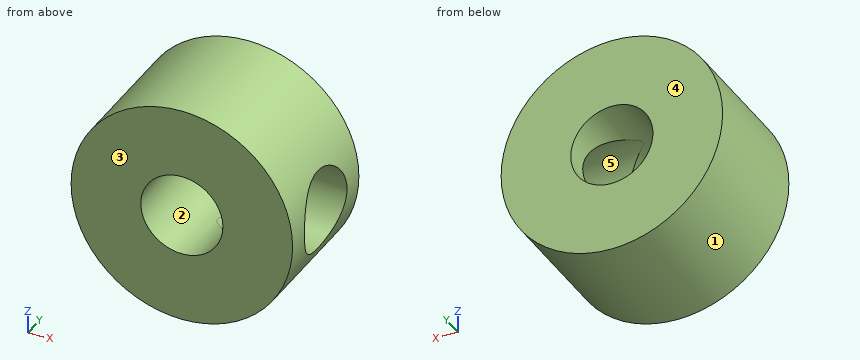
Autodesk Inventor part; units mm, degrees
ref_plane "Work Plane1" through (5.5182, 0, 0) normal (1, 0, 0) x (0, 1, 0)
ref_plane "XZ Plane" through (0, 0, 0) normal (0, 1, 0) x (-1, 0, 0)
ref_plane "XY Plane" through (0, 0, 0) normal (0, 0, 1) x (1, 0, 0)
sketch "Sketch1" plane through (0, 0, 0) normal (0, 1, 0) x (-1, 0, 0)
  circle A0 centre (0, 0) radius 5.5182
  dimension "d0" = 11.0363
extrude "Extrusion1" add sketch "Sketch1" along normal blind 6.3779
sketch "Sketch2" plane through (0, 6.3779, 0) normal (0, 1, 0) x (1, 0, 0)
  circle A0 centre (0, 0) radius 2.046
  dimension "d3" = 4.0919
extrude "Extrusion2" cut sketch "Sketch2" against normal blind 11.1125
ref_plane "Work Plane1" through (5.5182, 0, 0) normal (1, 0, 0) x (0, 1, 0)
sketch "Sketch3" plane through (5.5182, 0, 0) normal (1, 0, 0) x (0, 1, 0)
  line L0 (6.3779, -5.5182) -> (6.3779, 5.5182)
  line L1 (6.3779, 0) -> (0, 0)
  circle A0 centre (3.189, 0) radius 2.0472
  dimension "d6" = 4.0945
extrude "Extrusion3" cut sketch "Sketch3" against normal blind 5.3975
properties part number "Axle hub with no cricle thing"
The model under review builds one solid part; all positions refer to its coordinate system, in mm. Face numbers are marked on the shaded views. A direction names the side the tool comes from. Coordinates: 2 decimals unless noted, no trailing zeros. Write each loop counter-clockwise with the first axis right and the second up, starting at its lowest first coordinate (ties: lowest second). Pieces come first, ordered by that corner, then holes. Notation, with made-up numbers: (-4, 38) - (45, 38) arc R24 ccw to (45, 74) - close; hole circle Ø2 at (-33.5, 58.5). An arc over 180 degrees is marked (long way). Answer as CSV lines item,"result".
(1) We need section B-B (x = 1.5). Give the boundary of the cut face in (y, z), plus the area to 3 significant figures.
Data:
outline,"(0, -5.31) - (6.38, -5.31) - (6.38, -1.39) - (4.69, -1.39) arc R2.05 cw to (1.69, -1.39) - (0, -1.39) - close; (0, 1.39) - (1.69, 1.39) arc R2.05 cw to (4.69, 1.39) - (6.38, 1.39) - (6.38, 5.31) - (0, 5.31) - close"
area,"47.3 mm2"
(2) We need section C-C (y = 5.75). Give the boundary of the cut face in (x, z).
Data:
outline,"circle Ø11.04 at (0, 0); hole circle Ø4.09 at (0, 0)"
(3) Tool access review of the marked faces 4 and 5: name each direction out of +Z, -Z, +X, -X, +Y, -Y from which nothing blocks a thin tool from reaching the whole face with its end or side.
Data:
face 4,"+Z, -Z, +X, -X, +Y"
face 5,"+X"
(4) We need section D-D (x = 4). Give the boundary of the cut face in (y, z), plus the area to 3 significant figures.
Data:
outline,"(0, -3.8) - (6.38, -3.8) - (6.38, 3.8) - (0, 3.8) - close; hole circle Ø4.09 at (3.19, 0)"
area,"35.3 mm2"
(5) Clearance check with flat-ended pins moving along their axes: pin 1 Ø1 at (y, z) = (4, 3.5) entering from -X; pin 2 Ø1 at (x, y) = (3, 3.5) entering from -Z. State where each tip first meets the part, or that it passes through.
Data:
pin 1,"stops at x = -4.63"
pin 2,"stops at z = -4.92"
(6) For line 1 along Z through (x, y) = (0, 4.75); line 2 along Y through (x, z) = (4, 0); line 3 along X through (y, z) = (1, -0.75), list the stretches that pass through material, from the lowest coordinate up. Write a range as [from, to].
Data:
line 1,"z = [-5.52, -2.05], [2.05, 5.52]"
line 2,"y = [0, 1.14], [5.24, 6.38]"
line 3,"x = [-5.47, -1.9], [1.9, 5.47]"
(7) We need section A-A (z = 0). Give the boundary of the cut face in (x, y).
Data:
outline,"(-5.52, 0) - (-2.05, 0) - (-2.05, 6.38) - (-5.52, 6.38) - close; (2.05, 0) - (5.52, 0) - (5.52, 1.14) - (2.05, 1.14) - close; (2.05, 5.24) - (5.52, 5.24) - (5.52, 6.38) - (2.05, 6.38) - close"
(8) Mouldability with a two-part tool opening along X and no side actions: class the marked faces 1, 2 and 3 as pulls with the +X half, pulls with the -X half, needs draft (parallel to the pull), parting line crosses it, or undercut.
Data:
face 1,"parting line crosses it"
face 2,"undercut"
face 3,"needs draft"
